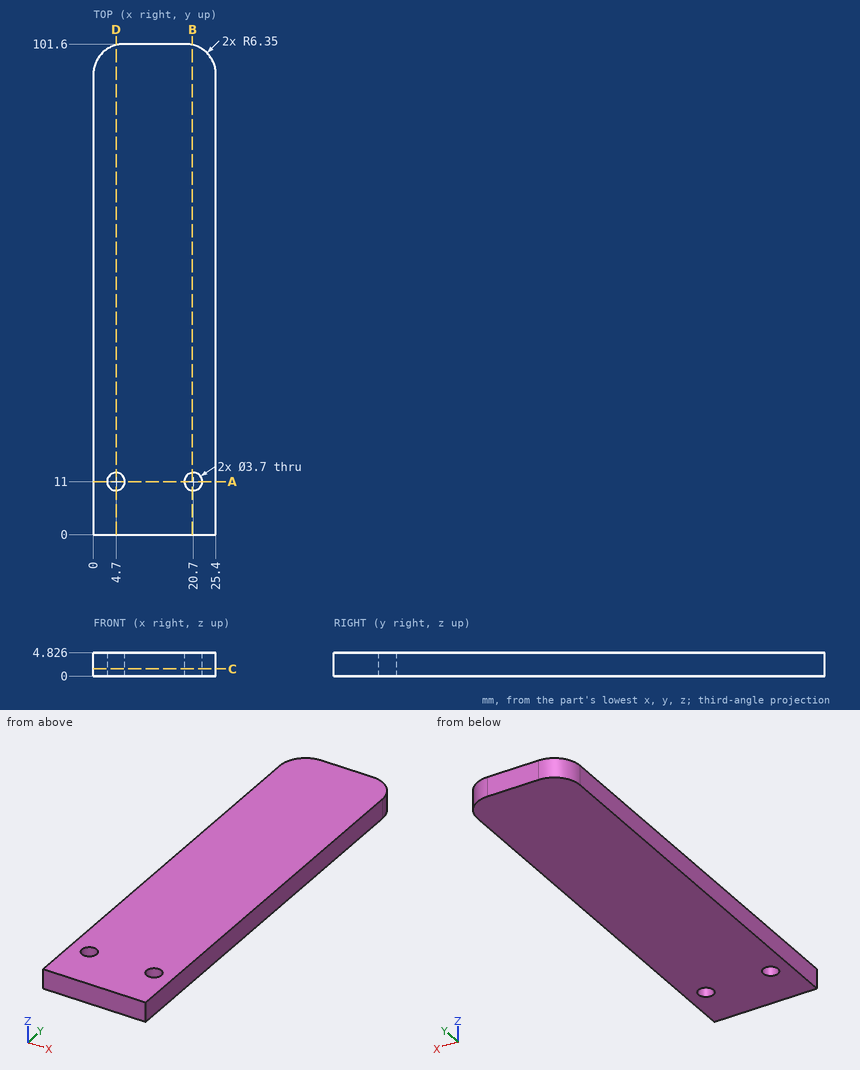
Part print with two shaded views. Sizes in mm from the minimum x, y, z corner. Coordinates: 2 decimals unless noted, no trailing zeros. Loops run counter-clockwise (first coordinate to the right, second up) from the corner with the lowest first, then second, coordinate; pieces in that order, holes last. Notation, with made-up numbers: (15.25, 67) -> (20.25, 67) arc R22 cw to (20.25, 76) -> close; hole circle Ø11 at (-39.75, 4). An arc over 180 degrees is marked (long way). Answer as a JSON object with one key per item and string values.
Q1. Probe probe 1 along Y at (x, z) = (6, 4.55); probe 2 along Y at (x, z) = (20.7, 2.8); probe 3 along Y at (x, z) = (1, 4.5). List the from-to ranges inside material, lowest first.
Report:
{"probe 1": "y = 0 to 9.68, 12.32 to 101.59", "probe 2": "y = 0 to 9.15, 12.85 to 101.38", "probe 3": "y = 0 to 98.67"}
Q2. Cut at A-A (y = 11). List the corners of the cut face in (x, z).
Report:
{"outline": "(0, 0) -> (2.85, 0) -> (2.85, 4.83) -> (0, 4.83) -> close; (6.55, 0) -> (18.85, 0) -> (18.85, 4.83) -> (6.55, 4.83) -> close; (22.55, 0) -> (25.4, 0) -> (25.4, 4.83) -> (22.55, 4.83) -> close"}
Q3. Cut at C-C (z = 1.45). List the corners of the cut face in (x, y), and give its area (3 significant figures).
Report:
{"outline": "(0, 0) -> (25.4, 0) -> (25.4, 95.25) arc R6.35 ccw to (19.05, 101.6) -> (6.35, 101.6) arc R6.35 ccw to (0, 95.25) -> close; hole circle Ø3.7 at (4.7, 11); hole circle Ø3.7 at (20.7, 11)", "area": "2,540 mm2"}
Q4. Cut at D-D (x = 4.7). List the corners of the cut face in (y, z), and give its area (3 significant figures).
Report:
{"outline": "(0, 0) -> (9.15, 0) -> (9.15, 4.83) -> (0, 4.83) -> close; (12.85, 0) -> (101.38, 0) -> (101.38, 4.83) -> (12.85, 4.83) -> close", "area": "471 mm2"}
Q5. Cut at B-B (x = 20.5). List the corners of the cut face in (y, z), and give its area (3 significant figures).
Report:
{"outline": "(0, 0) -> (9.16, 0) -> (9.16, 4.83) -> (0, 4.83) -> close; (12.84, 0) -> (101.43, 0) -> (101.43, 4.83) -> (12.84, 4.83) -> close", "area": "472 mm2"}
Q6. Flat gauge pins, fed straight in: P1, Ø2, axis at x = 21, z = 2, coming from the +Y side; P2, Ø3.5, axis at x = 4.7, y = 11, coming from the -Z side. Where does each tip first touch, or does it go through?
Report:
{"P1": "stops at y = 101.53", "P2": "passes through"}
